The listing builds one solid part. Answer for the finished solid, in the listing's coordinates (mm). Face numbers are marked on the shaded views. A direction names the side the tool comes from. Coordinates: 2 decimals unless noted, no trailing zeros. Order: outer loops, then holes, each group sorted by start corner. A loop starts at its lowest first (then second) coordinate and runs counter-clockwise, first axis right, second up. Notation, with made-up numbers: (44, 12.25) -> (50, 12.25) arc R19 cw to (50, 22.25) -> close; hole circle Ø2 at (51.25, 67.25). An arc over 180 degrees is marked (long way). One line per question, with ' | ' between items.
from build123d import *

# Parameters (mm, degrees)
SKETCH1_R           = 2
BOSS_EXTRUDE1_DEPTH = 15
SKETCH2_W           = 10
SKETCH2_H           = 23.787832066
CUT_EXTRUDE1_DEPTH  = 33.511536414
SKETCH5_W           = 7
SKETCH5_H           = 6
BOSS_EXTRUDE3_DEPTH = 2
SKETCH3_R           = 1.25
CUT_EXTRUDE2_DEPTH  = 33.511536414
SKETCH4_W           = 24
SKETCH4_H           = 3
BOSS_EXTRUDE2_DEPTH = 5
CUT_EXTRUDE3_DEPTH  = 31.528675045


with BuildPart() as part:
    # Sketch1 → Boss-Extrude1 (new body)
    with BuildSketch(Plane.XY):
        with BuildLine():
            Line((0, 0), (24, 0))
            Line((24, 0), (24, 3))
            Line((24, 3), (15.166426501, 14.444124223))
            ThreePointArc((15.166426501, 14.444124223), (12, 16), (8.833573499, 14.444124223))
            Line((8.833573499, 14.444124223), (0, 3))
            Line((0, 3), (0, 0))
        make_face()
        with Locations((12, 12)):
            Circle(SKETCH1_R, mode=Mode.SUBTRACT)
    extrude(amount=BOSS_EXTRUDE1_DEPTH)

    # Sketch2 → Cut-Extrude1 (cut, through all)
    with BuildSketch(Plane(origin=(24, 0, 0), x_dir=(0, 0, -1), z_dir=(1, 0, 0))):
        with Locations((-5, 14.893916033)):
            Rectangle(SKETCH2_W, SKETCH2_H)
    extrude(amount=-CUT_EXTRUDE1_DEPTH, mode=Mode.SUBTRACT)

    # Sketch5 → Boss-Extrude3 (add)
    with BuildSketch(Plane(origin=(0, 3, 0), x_dir=(-1, 0, 0), z_dir=(0, 1, 0))):
        with Locations((-20.5, 7)):
            Rectangle(SKETCH5_W, SKETCH5_H)
        with Locations((-3.5, 7)):
            Rectangle(SKETCH5_W, SKETCH5_H)
    extrude(amount=BOSS_EXTRUDE3_DEPTH)

    # Sketch3 → Cut-Extrude2 (cut, through all)
    with BuildSketch(Plane.XZ):
        with Locations((4, 7)):
            Circle(SKETCH3_R)
        with Locations((20, 7)):
            Circle(SKETCH3_R)
    extrude(amount=-CUT_EXTRUDE2_DEPTH, mode=Mode.SUBTRACT)

    # Sketch4 → Boss-Extrude2 (add)
    with BuildSketch(Plane(origin=(0, 14, 15), x_dir=(1, 0, 0), z_dir=(0, 0, -1))):
        with Locations((12, 12.5)):
            Rectangle(SKETCH4_W, SKETCH4_H)
    extrude(amount=-BOSS_EXTRUDE2_DEPTH)

    # Sketch6 → Cut-Extrude3 (cut, through all)
    with BuildSketch(Plane.XY.offset(10)):
        Polygon((0, 5), (0, 3), (1.543774487, 5), align=None)
        Polygon((24, 5), (22.456225513, 5), (24, 3), align=None)
    extrude(amount=-CUT_EXTRUDE3_DEPTH, mode=Mode.SUBTRACT)


solid = part.part
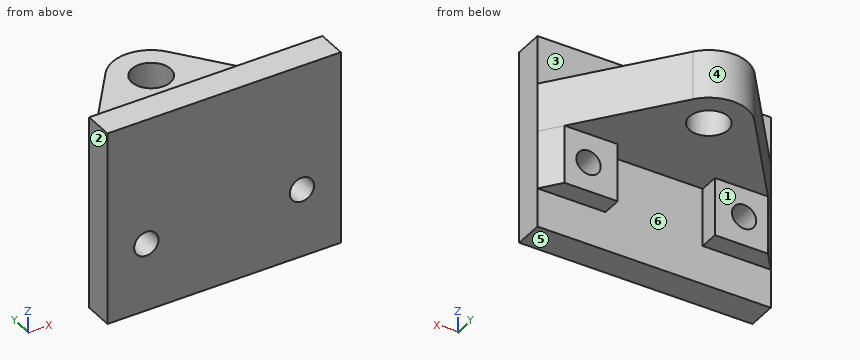
Item 1: Section C-C, the plane y = 12.75 is taken. Give the vertices of the cut face in (x, z), plus the area to 3 significant figures.
Computed values:
outline: (7.53, 10) -> (10.15, 10) -> (10.15, 15) -> (7.53, 15) -> close; (13.85, 10) -> (16.47, 10) -> (16.47, 15) -> (13.85, 15) -> close | area: 26.2 mm^2
Item 2: Determine the mould class of the marked faces 4, 5 and 6 for opening direction X: pulls with the +X half, pulls with the -X half, needs draft (parallel to the pull), parting line crosses it, or undercut.
Computed values:
face 4: parting line crosses it | face 5: needs draft | face 6: undercut
Item 3: Each of these flat-tipped pins is pushed along its axis until it touches: pin 1 Ø4 at (x, y) = (8.5, 9.5) entering from -Z; pin 2 Ø0.6 at (y, z) = (4.5, 6.5) entering from -X; pin 3 Ø6 at (x, z) = (16.5, 3.5) entering from +Y; pin 4 Ø2 at (x, z) = (20, 7) entering from -Y. Where does it stop, or does it pass through?
Computed values:
pin 1: stops at z = 10 | pin 2: stops at x = 0.93 | pin 3: stops at y = 5 | pin 4: passes through
Item 4: Section D-D, the plane z = 7 is taken. Give the vertices of the cut face in (x, y), plus the area to 3 significant figures.
Computed values:
outline: (0, 0) -> (2.75, 0) -> (2.75, 5) -> (1.54, 5) -> (0, 3) -> close; (5.25, 0) -> (18.75, 0) -> (18.75, 5) -> (17, 5) -> (17, 3) -> (7, 3) -> (7, 5) -> (5.25, 5) -> close; (21.25, 0) -> (24, 0) -> (24, 3) -> (22.46, 5) -> (21.25, 5) -> close | area: 71.9 mm^2
Item 5: For the marked faces 1, 2 and 3, determine the directions among +Z, -Z, +X, -X, +Y, -Y from which every point of the face is accessible in a straight line to the end or side of a thin tool.
Computed values:
face 1: -Z, +X, -X, +Y | face 2: +Z, -Z, -X, +Y, -Y | face 3: +Z, +X, -X, +Y
Item 6: Find the intervals of material crossed by L1, parallel to Z at x = 4, y = 1.45; L2, parallel to Z at x = 4, y = 3.75; L3, parallel to Y at x = 12, z = 12.7, in increasing order.
Computed values:
L1: z = 0 to 5.75, 8.25 to 20 | L2: z = 4 to 5.75, 8.25 to 15 | L3: y = 0 to 10, 14 to 16
Item 7: Section B-B, the plane z = 10.5 is taken. Give the vertices of the cut face in (x, y), plus the area to 3 significant figures.
Computed values:
outline: (0, 0) -> (24, 0) -> (24, 3) -> (15.17, 14.44) arc R4 ccw to (8.83, 14.44) -> (0, 3) -> close; hole circle Ø4 at (12, 12) | area: 240 mm^2
Item 8: Section A-A, the plane x = 12 is taken. Give the vertices of the cut face in (y, z), plus the area to 3 significant figures.
Computed values:
outline: (0, 0) -> (3, 0) -> (3, 10) -> (10, 10) -> (10, 15) -> (3, 15) -> (3, 20) -> (0, 20) -> close; (14, 10) -> (16, 10) -> (16, 15) -> (14, 15) -> close | area: 105 mm^2
